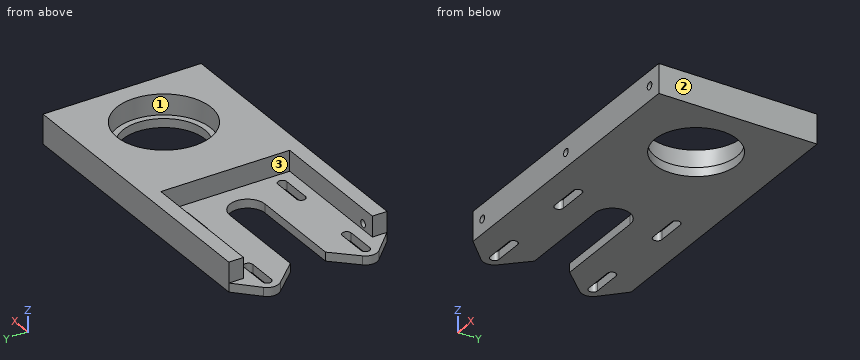
Autodesk Inventor part; units mm, degrees
ref_plane "РабПлоскость1" through (-50, 0, 0) normal (0, 1, 0) x (1, 0, 0)
ref_plane "YZ Plane" through (0, 0, 0) normal (1, 0, 0) x (0, 1, 0)
ref_plane "XZ Plane" through (0, 0, 0) normal (0, 1, 0) x (-1, 0, 0)
sketch "Эскиз1" plane through (0, 0, 0) normal (0, 0, 1) x (1, 0, 0)
  line L0 (50, -27) -> (-50, -27)
  line L1 (-50, -27) -> (-50, 27)
  line L2 (-50, 27) -> (50, 27)
  line L3 (50, 27) -> (50, -27)
  line L4 (50, -27) -> (-50, 27) construction
  line L5 (-50, -27) -> (50, 27) construction
  circle A0 centre (27.5, 0) radius 16.05
  point P0 (0, 0)
  point P1 (0, 0)
  dimension "d0" = 100
  dimension "d1" = 54
  dimension "d2" = 32.1
  dimension "d3" = 22.5
extrude "Выдавливание1" add sketch "Эскиз1" along normal blind 10
sketch "Эскиз2" plane through (0, 0, 0) normal (0, 0, -1) x (-1, 0, 0)
  circle A0 centre (-27.5, 0) radius 16.05
  circle A1 centre (-27.5, 0) radius 14
  point P0 (0, 0)
  dimension "d6" = 28
extrude "Выдавливание2" add sketch "Эскиз2" against normal blind 3
sketch "Эскиз3" plane through (0, 0, 0) normal (0, 0, -1) x (-1, 0, 0)
  circle A0 centre (-27.5, 0) radius 14
  circle A1 centre (17.5, 0) radius 6
  line L0 (17.5, 6) -> (50, 6)
  line L1 (50, -27) -> (50, 27)
  line L2 (17.5, -6) -> (50, -6)
  line L3 (50, -6) -> (50, 6)
  point P0 (0, 0)
  dimension "d9" = 12
  dimension "d10" = 45
extrude "Выдавливание3" cut sketch "Эскиз3" against normal blind 10 contours A1 | A1 L0 L1 L2
sketch "Эскиз4" plane through (0, 0, 10) normal (0, 0, 1) x (1, 0, 0)
  line L0 (-49.5, 22) -> (-5.5, 22)
  line L1 (-5.5, 22) -> (-5.5, -22)
  line L2 (-5.5, -22) -> (-49.5, -22)
  line L3 (-49.5, -22) -> (-49.5, 22)
  line L4 (-49.5, 22) -> (-5.5, -22) construction
  line L5 (-5.5, 22) -> (-49.5, -22) construction
  arc A0 (-17.5, -6) -> (-17.5, 6) centre (-17.5, 0) ccw
  line L6 (-49.5, -22) -> (-62.5164, -22)
  line L7 (-62.5164, -22) -> (-62.5164, 22)
  line L8 (-62.5164, 22) -> (-49.5, 22)
  line L9 (-49.5, 22) -> (-49.5, -22)
  point P0 (0, 0)
  point P1 (-27.5, 0)
  point P2 (-27.5, 0)
  dimension "d13" = 44
  dimension "d14" = 44
  dimension "d15" = 10
  dimension "d16" = 44
extrude "Выдавливание4" cut sketch "Эскиз4" against normal blind 7
sketch "Эскиз8" plane through (-50, -27, 10) normal (0, -1, 0) x (1, 0, 0)
  circle A0 centre (95, -5) radius 1.25
  circle A1 centre (50, -5) radius 1.25
  circle A2 centre (5, -5) radius 1.25
  line L0 (100, -10) -> (100, 0)
  line L1 (0, -10) -> (0, 0)
  line L2 (100, -10) -> (0, -10)
  point P0 (50, -10)
  point P1 (100, -5)
  point P2 (0, -7)
  point P3 (50, -10)
  dimension "d44" = 2.5
  dimension "d45" = 2.5
  dimension "d46" = 2.5
  dimension "d47" = 5
  dimension "d48" = 5
extrude "Выдавливание9" cut sketch "Эскиз8" against normal up to surface (5 mm away)
sketch "Эскиз9" plane through (0, 0, 0) normal (0, 0, -1) x (-1, 0, 0)
  circle A0 centre (10.0218, 16.95) radius 1.5
  circle A1 centre (44.6782, 16.95) radius 1.5
  circle A2 centre (44.6782, -16.65) radius 1.5
  circle A3 centre (10.0218, -16.65) radius 1.5
  line L0 (-50, 27) -> (50, 27)
  line L1 (-50, -27) -> (-50, 27)
  line L2 (50, -27) -> (-50, -27)
  line L3 (50, -22) -> (50, -6)
  line L4 (50, 6) -> (50, 22)
  point P0 (0, 0)
  dimension "d75" = 10.05
  dimension "d76" = 60.0218
  dimension "d77" = 3
  dimension "d78" = 10.05
  dimension "d79" = 10.35
  dimension "d80" = 10.35
  dimension "d82" = 5.3218
  dimension "d83" = 3
  dimension "d84" = 3
  dimension "d85" = 3
extrude "Выдавливание10" cut sketch "Эскиз9" against normal blind 10
sketch "Эскиз10" plane through (0, 0, 0) normal (0, 0, -1) x (-1, 0, 0)
  circle A0 centre (10.0218, 16.95) radius 1.5
  line L0 (10.0218, 18.45) -> (20.0218, 18.45)
  line L1 (10.0218, 15.45) -> (20.0218, 15.45)
  circle A1 centre (20.0218, 16.95) radius 1.5
  circle A2 centre (10.0218, -16.65) radius 1.5
  line L2 (10.0218, -15.15) -> (20.0218, -15.15)
  line L3 (10.0218, -18.15) -> (20.0218, -18.15)
  circle A3 centre (20.0218, -16.65) radius 1.5
  line L4 (20.0218, 18.45) -> (20.0218, 15.45)
  line L5 (10.0218, 18.45) -> (10.0218, 15.45)
  line L6 (10.0218, -15.15) -> (10.0218, -18.15)
  line L7 (20.0218, -15.15) -> (20.0218, -18.15)
  point P0 (0, 0)
  dimension "d53" = 10
  dimension "d54" = 10
  dimension "d55" = 10
  dimension "d56" = 10
extrude "Выдавливание11" cut sketch "Эскиз10" against normal blind 10 contours A0 L5 | A0 L0 A1 L1 | L4 A1 | A1 L4 | A2 L2 A3 L3 | L7 A3 | A3 L7 picked at (10.3335, 17.3409)
sketch "Эскиз11" plane through (0, 0, 0) normal (0, 0, -1) x (-1, 0, 0)
  line L0 (-50, 27) -> (50, 27)
  line L1 (50, 6) -> (50, 27)
  line L2 (50, 27) -> (50, 6)
  circle A0 centre (44.6782, 16.95) radius 1.5
  line L3 (44.6782, 18.45) -> (54.6782, 18.45)
  line L4 (54.6782, 18.45) -> (54.6782, 15.45)
  line L5 (54.6782, 15.45) -> (44.6782, 15.45)
  arc A1 (54.6782, 15.45) -> (54.6782, 18.45) centre (54.6782, 16.95) ccw
  arc A2 (57.6149, 14.2342) -> (57.4511, 19.8328) centre (54.6782, 16.95) ccw
  line L6 (50, 27) -> (57.4511, 19.8328)
  line L7 (50, 6) -> (57.6149, 14.2342)
  point P0 (0, 0)
  point P1 (50, 16.5)
  dimension "d60" = 10
  dimension "d61" = 3
  dimension "d62" = 8
extrude "Выдавливание12" add sketch "Эскиз11" against normal up to surface (3 mm away) contours L1 L5 A1 L3 L6 A2 L7 | L1 L3 L4 L5
extrude "Выдавливание13" cut sketch "Эскиз11" against normal blind 10 contours L5 A0 L3 L1 | L1 L3 L4 L5
ref_plane "РабПлоскость1" through (-50, 0, 0) normal (0, 1, 0) x (1, 0, 0)
sketch "Эскиз12" plane through (0, 0, 0) normal (0, 0, -1) x (-1, 0, 0)
  line L0 (50, -6) -> (17.5, -6)
  line L1 (50, -22) -> (50, -27)
  line L2 (50, -6) -> (50, -27)
  circle A0 centre (44.6782, -16.65) radius 1.5
  line L3 (44.6782, -15.15) -> (54.6782, -15.15)
  line L4 (54.6782, -18.15) -> (54.6782, -15.15)
  line L5 (54.6782, -18.15) -> (44.6782, -18.15)
  circle A1 centre (54.6782, -16.65) radius 1.5
  arc A2 (57.5094, -19.4756) -> (57.5639, -13.8801) centre (54.6782, -16.65) ccw
  line L6 (50, -22) -> (50, -6)
  line L7 (50, -6) -> (57.5639, -13.8801)
  line L8 (50, -27) -> (57.5094, -19.4756)
  point P0 (0, 0)
  dimension "d67" = 10
  dimension "d68" = 10
  dimension "d69" = 3
  dimension "d70" = 8
extrude "Выдавливание14" add sketch "Эскиз12" against normal up to surface (3 mm away) contours L2 L5 A1 L3 L7 A2 L8 L1 | L2 L3 A1 L5
extrude "Выдавливание15" cut sketch "Эскиз12" against normal blind 10 contours L5 A0 L3 L2 | L2 L3 A1 L5 | A1 L4 | L4 A1
equation "\"d44\" = d45"
equation "\"d45\" = d46"
properties part number "крепление подшипникового блока левая часть"
Work out the finished part from the listing and answer in its coordinate system (mm). Face numbers are marked on the shaded views. A direction names the side the tool comes from. Coordinates: 2 decimals unless noted, no trailing zeros. Write each loop counter-clockwise with the first axis right and the second up, starting at its lowest first coordinate (ties: lowest second). Pieces come first, ordered by that corner, then holes. Notation, with made-up numbers: M 48.25,27 L 101.25,27 A14 cw 101.25,37 Z; hole C 79.5,-32.5 d10. An arc over 180 degrees is marked long. Answer as CSV lines item,"result". Start each with the question number.
Item 1: Flat-ended cylindrical pins translate along their axes: P1, Ø0.9, axis at x = -52, z = 1, coming from the -Y side; P2, Ø10, axis at x = 34, y = -11, coming from the +Z side; P3, Ø2.5, axis at y = -25.5, z = 5.5, coming from the -X side; P4, Ø2.5, axis at x = -51.5, z = 2, coming from the -Y side. Find the tip coordinate at first contact, or state that the pin passes through.
Item 2: Section C-C on z = 8.5 is taken. Write down the section's boundary in (x, y).
Item 3: Section B-B on y = 0 is taken. Write down the section's boundary in (x, z), and give its area (3 significant figures).
Item 4: Section A-A on x = -23 is taken. Write down the section's boundary in (y, z), and give its area (3 significant figures).
Item 5: Section D-D on x = 27.5 is taken. Write down the section's boundary in (y, z), and give its area (3 significant figures).
Item 6: A tool of negligible diameter and unlimited length cuts with its end or side. For the marked faces 1, 2 and 3, from which of +Z, -Z, +X, -X, +Y, -Y can it reach the whole face along a straight path? Write none if from no direction.
Item 7: Consider L1, parallel to Y at x = -17, z = 2.5; L2, parallel to Z at x = 0, y = -25; L3, parallel to Y at x = -7.5, z = 9. Determine where each line is inside the solid, lowest interval first.
Checks:
1,P1,"stops at y = -25.45"
1,P2,"stops at z = 10"
1,P3,"stops at x = -50"
1,P4,"stops at y = -26.75"
2,outline,"M -50,-27 L 50,-27 L 50,27 L -50,27 L -50,22 L -5.5,22 L -5.5,-22 L -50,-22 Z; hole C 27.5,0 d32.1"
3,outline,"M -11.5,0 L 13.5,0 L 13.5,3 L 11.45,3 L 11.45,10 L -5.5,10 L -5.5,3 L -11.5,3 Z; M 41.5,0 L 50,0 L 50,10 L 43.55,10 L 43.55,3 L 41.5,3 Z"
3,area,"264 mm²"
4,outline,"M -27,0 L -6,0 L -6,3 L -22,3 L -22,10 L -27,10 Z; M 6,0 L 27,0 L 27,10 L 22,10 L 22,3 L 6,3 Z"
4,area,"196 mm²"
5,outline,"M -27,0 L -14,0 L -14,3 L -16.05,3 L -16.05,10 L -27,10 Z; M 14,0 L 27,0 L 27,10 L 16.05,10 L 16.05,3 L 14,3 Z"
5,area,"231 mm²"
6,face 1,"+Z"
6,face 2,"+Z, -Z, +X, +Y, -Y"
6,face 3,"+Z, -X"
7,L1,"y = -27 to -18.15, -15.15 to -5.98, 5.98 to 15.45, 18.45 to 27"
7,L2,"z = 0 to 3.75, 6.25 to 10"
7,L3,"y = -27 to -22, 22 to 27"
